Part model, mm, in its own coordinate system. Face numbers are marked on the shaded views. A direction names the side the tool comes from. Coordinates: 2 decimals unless noted, no trailing zeros. Order: outer loops, then holes, each group sorted by start corner. A loop starts at its lowest first (then second) coordinate and runs counter-clockwise, first axis right, second up.
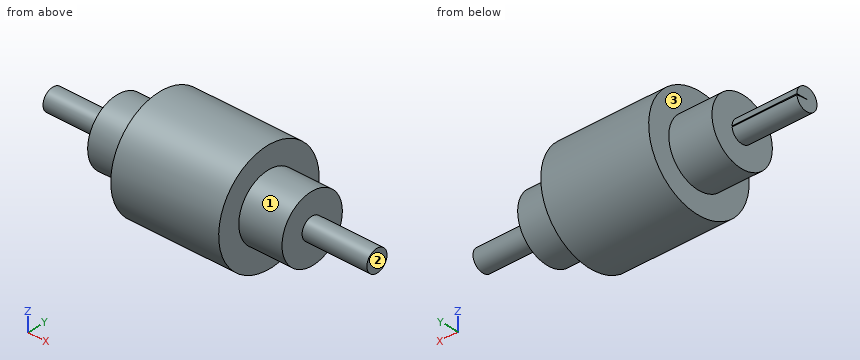
```python
from build123d import *

# Parameters (mm, degrees)
REVOLVE_THIN4_START = -152.206983034
REVOLVE_THIN4_DEPTH = 60
SKETCH1_7_W         = 60
SKETCH1_7_H         = 10


# Read off the part's stored shape, not the designer's step: Revolve-Thin4
with BuildPart() as part:
    # Revolve-Thin4 outline → Revolve-Thin4 (new body)
    with BuildSketch(Plane.YZ.offset(REVOLVE_THIN4_START)):
        with BuildLine():
            ThreePointArc((10, 0), (-9.990482216, 0.436193872), (9.961946981, -0.871557427))
            Line((9.961946981, -0.871557427), (0, 0))
            Line((0, 0), (10, 0))
        make_face()
    extrude(amount=REVOLVE_THIN4_DEPTH)

    # Sketch1<7> → Revolve2 (revolve)
    with BuildSketch(Plane.XY, mode=Mode.PRIVATE) as revolve2_sk:
        Polygon((-92.206983034, 10), (-92.206983034, 0), (-52.206983034, 0), (-52.206983034, 30), (-92.206983034, 30), align=None)
        Polygon((-52.206983034, 30), (-52.206983034, 0), (47.793016966, 0), (47.793016966, 30), (47.793016966, 50), (-52.206983034, 50), align=None)
        Polygon((47.793016966, 30), (47.793016966, 0), (87.793016966, 0), (87.793016966, 10), (87.793016966, 30), align=None)
        with Locations((117.793016966, 5)):
            Rectangle(SKETCH1_7_W, SKETCH1_7_H)
    revolve(revolve2_sk.sketch.rotate(Axis((-163.404059647, 0, 0), (1, 0, 0)), 90), axis=Axis((-163.404059647, 0, 0), (1, 0, 0)))


solid = part.part
```
(1) Drop flat-ended pins along their axis: pin 1 (12 mm diameter, centred on x = -121, z = 3, fed in from +Y); pin 2 (1.5 mm diameter, centred on y = -22.5, z = -6.5, fed in from -X); pin 3 (3 mm diameter, centred on x = -34.5, y = 36, fed in from +Z). Give the stop position or say it passes through.
(2) Slice it at D-D, the plane x = 124.5. Give the cut face in (y, z), then the cut area to 3 significant figures.
(3) Slice it at C-C, the plane x = 64. Give the cut face in (y, z).
(4) Slice it at B-B, the plane z = -23.5. Give the cut face in (x, y).
(5) Tool access for the marked faces 1, 2 and 3: list every direction of +Z, -Z, +X, -X, +Y, -Y with a clear straight run to the whole face (end or side of a thin tool).
(6) Slice it at A-A, the plane y = -24. Give the cut face in (x, z).
(7) Probe line 1 (X direction, y = 45, z = -15); line 2 (X direction, y = 28.5, z = -8.5); line 3 (Y direction, x = -21, z = 10). List the from-to ranges inside material, lowest first.
Here are the results:
1. pin 1: stops at y = 10
1. pin 2: stops at x = -92.21
1. pin 3: stops at z = 36.19
2. outline: circle Ø20 at (0, 0)
2. area: 314 mm2
3. outline: circle Ø60 at (0, 0)
4. outline: (-92.21, -18.65) - (-52.21, -18.65) - (-52.21, -44.13) - (47.79, -44.13) - (47.79, -18.65) - (87.79, -18.65) - (87.79, 18.65) - (47.79, 18.65) - (47.79, 44.13) - (-52.21, 44.13) - (-52.21, 18.65) - (-92.21, 18.65) - close
5. face 1: +X
5. face 2: +Z, -Z, +X, +Y, -Y
5. face 3: -X
6. outline: (-92.21, -18) - (-52.21, -18) - (-52.21, -43.86) - (47.79, -43.86) - (47.79, -18) - (87.79, -18) - (87.79, 18) - (47.79, 18) - (47.79, 43.86) - (-52.21, 43.86) - (-52.21, 18) - (-92.21, 18) - close
7. line 1: x = -52.21 to 47.79
7. line 2: x = -92.21 to 87.79
7. line 3: y = -48.99 to 48.99
